```python
from build123d import *

# Parameters (mm, degrees)
F0_W     = 59
F0_H     = 14
F0_R     = 2.5
F0_W_2   = 16.1
F0_H_2   = 8.8
F1_DEPTH = 5.5
F2_DEPTH = 18.5
F3_R     = 4.2
F4_R     = 2
F5_R     = 1
F7_DEPTH = 25
F8_R     = 1.59999


# Not quite as in the source:
# - a fillet or chamfer is up to 0.001 mm smaller than in the source, because OpenCascade refuses the exact size


with BuildPart() as f1:
    # F0 (on Right) → F1 (new body)
    with BuildSketch(Plane.YZ):
        Rectangle(F0_W, F0_H)
        with Locations((-25, 0)):
            Circle(F0_R, mode=Mode.SUBTRACT)
        Rectangle(F0_W_2, F0_H_2, mode=Mode.SUBTRACT)
        with Locations((25, 0)):
            Circle(F0_R, mode=Mode.SUBTRACT)
    extrude(amount=F1_DEPTH)

    # F0 (on Right) → F2 (join)
    with BuildSketch(Plane.YZ):
        Rectangle(F0_W_2, F0_H_2)
        Circle(F0_R, mode=Mode.SUBTRACT)
        Circle(F0_R)
    extrude(amount=F2_DEPTH)

    # F3
    f3_edges = [f1.edges().sort_by_distance(p)[0] for p in [
        (18.5, 0, 4.4),
        (18.5, 0, -4.4),
    ]]
    fillet(f3_edges, radius=F3_R)

    # F4
    f4_edges = [f1.edges().sort_by_distance(p)[0] for p in [
        (2.75, 29.5, 7),
        (2.75, 29.5, -7),
        (2.75, -29.5, 7),
        (2.75, -29.5, -7),
    ]]
    fillet(f4_edges, radius=F4_R)

    # F5
    f5_edges = [f1.edges().sort_by_distance(p)[0] for p in [
        (5.5, 0, 7),
    ]]
    fillet(f5_edges, radius=F5_R)

    # F6 (on face) → F7 (cut)
    with BuildSketch(Plane.XZ.offset(8.05)):
        with BuildLine():
            Line((5.5, 2.125), (5.5, -2.125))
            Line((5.5, -2.125), (15, -2.125))
            ThreePointArc((15, -2.125), (17.125, 0), (15, 2.125))
            Line((15, 2.125), (5.5, 2.125))
        make_face()
    extrude(amount=-F7_DEPTH, mode=Mode.SUBTRACT)

    # F8 (radius 1.6 in the source; OpenCascade refuses exactly that, so slightly less here)
    f8_edges = [f1.edges().sort_by_distance(p)[0] for p in [
        (5.5, 0, 4.4),
        (5.5, 0, -4.4),
        (5.5, 0, -2.125),
        (5.5, 0, 2.125),
    ]]
    fillet(f8_edges, radius=F8_R)


solid = f1.part
```
The listing builds one solid part. Answer for the finished solid, in the listing's coordinates (mm). A direction names the side the tool comes from. Round coordinates to 2 decimals unless told otherwise and drop trailing zeros. Write each loop counter-clockwise with the first axis right and the second up, starting at its lowest first coordinate (ties: lowest second). Pieces come first, ordered by that corner, then holes. Notation, with made-up numbers: (79, -17.75) -> (94, -17.75) arc R20 cw to (94, 3.25) -> close; hole circle Ø7 at (26, 70.25). An arc over 180 degrees is marked (long way). Write item = value, one per line.
1) Section B-B on x = 9 is taken. Write down the section's boundary in (y, z) (3 decimals).
Check values:
outline = (-8.05, -4.4) -> (8.05, -4.4) -> (8.05, -2.125) -> (-8.05, -2.125) -> close; (-8.05, 2.125) -> (8.05, 2.125) -> (8.05, 4.4) -> (-8.05, 4.4) -> close
2) Section C-C on y = 25 is taken. Write down the section's boundary in (x, z), plus the area to 3 significant figures.
Check values:
outline = (0, -7) -> (4.5, -7) arc R1 ccw to (5.5, -6) -> (5.5, -2.5) -> (0, -2.5) -> close; (0, 2.5) -> (5.5, 2.5) -> (5.5, 6) arc R1 ccw to (4.5, 7) -> (0, 7) -> close
area = 49.1 mm²
3) Given pin 1 (6 mm diameter, centred on x = 10.5, z = 2, fed in from -Y); pin 2 (1.5 mm diameter, centred on y = -13.5, z = -5, fed in from -X); pin 3 (2.5 mm diameter, centred on x = 9.5, y = -2.5, fed in from -Z); pin 4 (2 mm diameter, centred on x = 15.5, z = 3.5, fed in from +Y), each flat-ended and moving along its own axis, determine where each tip first touches the part or whether it passes through.
Check values:
pin_1 = -8.05
pin_2 = 0
pin_3 = -4.4
pin_4 = 8.05
4) For a pull along X with two mould halves and no side action, classify faces 6 (the flat face through (2, 0, -7)), 7 (the flat face through (11, 0, 2.125)), 8 (the cylindrical face through (5.215, 0.385, 6.699)) as released by +X, released by -X, zero draft, split by the parting line, or undercut.
Check values:
face_6 = zero draft
face_7 = undercut
face_8 = released by +X
5) Section D-D on z = 1.5 is taken. Write down the section's boundary in (x, y), plus the area to 3 significant figures.
Check values:
outline = (0, -29.5) -> (4.5, -29.5) arc R1 ccw to (5.5, -28.5) -> (5.5, -27) -> (0, -27) -> close; (0, -23) -> (5.5, -23) -> (5.5, -8.05) -> (5.83, -8.05) -> (5.83, 8.05) -> (5.5, 8.05) -> (5.5, 23) -> (0, 23) -> close; (0, 27) -> (5.5, 27) -> (5.5, 28.5) arc R1 ccw to (4.5, 29.5) -> (0, 29.5) -> close; (16.51, -8.05) -> (18.29, -8.05) -> (18.29, 8.05) -> (16.51, 8.05) -> close
area = 314 mm²
6) Which of the six approach directions +Z, -Z, +X, -X, +Y, -Y give full straight-line access (tool end or side, diameter ignored) to faces 1 (the flat face through (11, 0, 4.4)), 2 (the flat face through (12, 8.05, 3)), 3 (the flat face through (11, 0, -4.4)), 4 (the flat face through (12, -8.05, 3)), 5 (the cylindrical face through (5.956, 0.113, 1.644))?
Check values:
face_1 = +Z, +X, +Y, -Y
face_2 = +Z, -Z, +X, +Y
face_3 = -Z, +X, +Y, -Y
face_4 = +Z, -Z, +X, -Y
face_5 = +Y, -Y
7) Straight lines are drawn through the part: line 1 along Z through (x, y) = (3.4, 25); line 2 along Z through (x, y) = (13.5, -7.5) (3 decimals); line 3 along Y through (x, z) = (2, 1). For each, find the intervals that lie inside material, in ascending order. Write a range as [from, to].
Check values:
line_1 = [-7, -2.5], [2.5, 7]
line_2 = [-4.4, -2.125], [2.125, 4.4]
line_3 = [-29.5, -27.29], [-22.71, 22.71], [27.29, 29.5]
